For this review, use the dimensioned drawing (mm, ordinates from the lowest corner) and the shaded views. A direction names the side the tool comes from. Coordinates: 2 decimals unless noted, no trailing zeros. Loops run counter-clockwise (first coordinate to the right, second up) from the corner with the lowest first, then second, coordinate; pieces in that order, holes last. Notation, with made-up numbers: M 38.25,28.5 L 46.25,28.5 A26 ccw 46.25,67.5 Z; hole C -28.5,56 d9. An arc over 180 degrees is marked long. Write each question's results on one line, items separated by ' | '. Start each with the question number.
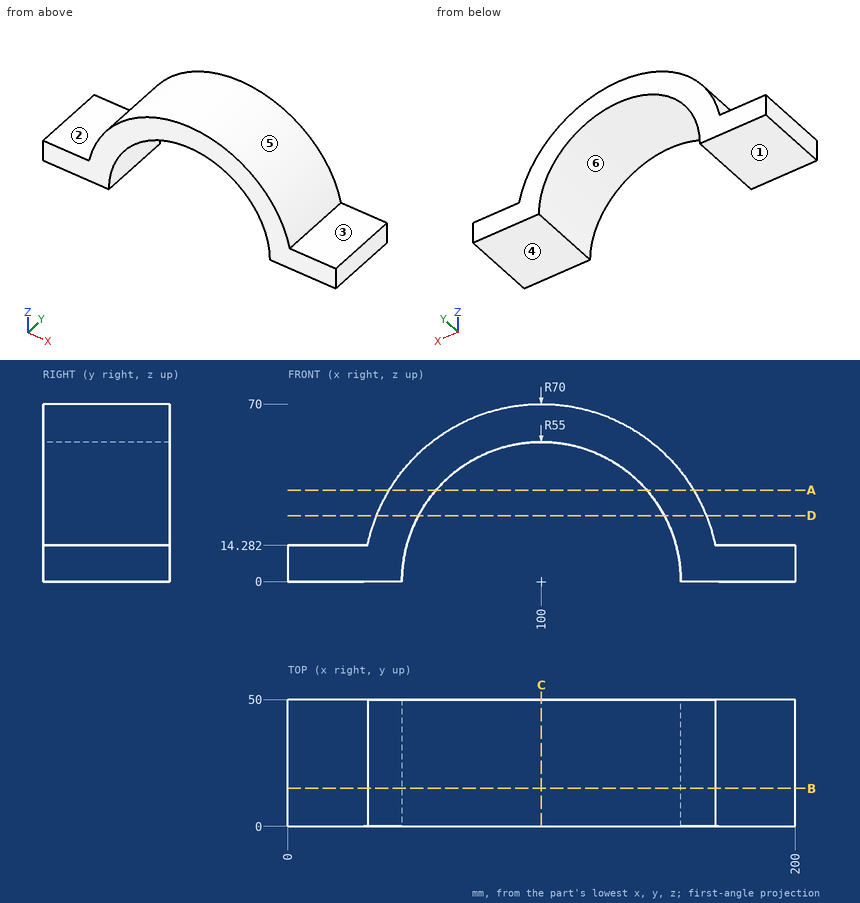
Q1. To check wall thickness, follow line 1 along Z through (x, y) = (19, 8); line 2 along X through (y, z) = (16.5, 51); line 3 along X through (y, z) = (11.5, 7). State the ranges of each line that lie inside material, in increasing order.
Q2. Take a section at D-D, the plane z = 26. Give the boundary of the cut face in (x, y).
Q3. Take a section at C-C, the plane x = 100. Give the boundary of the cut face in (y, z).
Q4. Take a section at A-A, the plane z = 36. Give the boundary of the cut face in (x, y).
Q5. Insertion check: P1, Ø4, axis at x = 139.5, y = 41, coming from the -Z side; P2, Ø15.5, axis at x = 11, y = 19.5, coming from the +Z side; P3, Ø10, axis at x = 128, y = 39, coming from the -Z side; P4, Ø10, axis at x = 45, z = 54, coming from the +Y side (1 decimal). Each pin has a flat end and moves straight along its axis. Give the tip position at first contact, or say it passes through.
Q6. For the marked faces 1, 2 and 3, list the 3-axis set-ups (+Z, -Z, +X, -X, +Y, -Y) from which the entire face can be reached by the end or side of a thin tool; tool diameter is ignored.
Q7. Take a section at B-B, the plane y = 15. Give the boundary of the cut face in (x, z), then the cut area to 3 significant figures.
Q8. The part is to be moulded in two halves that separate along X. For the marked faces 4, 5 and 6, say which applies: pulls with the +X half, pulls with the -X half, needs draft (parallel to the pull), parting line crosses it, or undercut.
Results:
1) line 1: 0 to 14.28 | line 2: 52.05 to 79.41, 120.59 to 147.95 | line 3: 0 to 45.45, 154.55 to 200
2) outline: M 35.01,0 L 51.53,0 L 51.53,50 L 35.01,50 Z; M 148.47,0 L 164.99,0 L 164.99,50 L 148.47,50 Z
3) outline: M 0,55 L 50,55 L 50,70 L 0,70 Z
4) outline: M 39.97,0 L 58.42,0 L 58.42,50 L 39.97,50 Z; M 141.58,0 L 160.03,0 L 160.03,50 L 141.58,50 Z
5) P1: z = 36.09 | P2: z = 14.28 | P3: z = 44 | P4: through
6) face 1: -Z, +X, -X, +Y, -Y | face 2: +Z, -X, +Y, -Y | face 3: +Z, +X, +Y, -Y
7) outline: M 0,0 L 45,0 A55 cw 155,0 L 200,0 L 200,14.28 L 168.53,14.28 A70 ccw 31.47,14.28 L 0,14.28 Z | area: 3,820 mm^2
8) face 4: needs draft | face 5: parting line crosses it | face 6: undercut
